Part model, mm, in its own coordinate system. Face numbers are marked on the shaded views. Coordinates: 2 decimals unless noted, no trailing zeros. Loops run counter-clockwise (first coordinate to the right, second up) from the corner with the lowest first, then second, coordinate; pieces in that order, holes last. Notation, with made-up numbers: (36.25, 81.25) - (52.25, 81.25) arc R23 cw to (52.25, 114.25) - close; hole circle Ø9 at (-22.5, 74). An arc over 180 degrees is marked (long way). Use a Markdown table: item, result. Add a question column.
1) Pull direction Z, two halves, no side cores. Call the marked faces 1, 2 and 3: +Z half, -Z half, draft (parallel to the pull), parting line (faces both ways), or undercut.
2) Drop flat-ended pins along their axis: P1, Ø1, axis at x = 0, z = 0, coming from the +Y side; P2, Ø1, axis at y = -4, z = -1, coming from the -X side; P3, Ø2, axis at x = -0.5, y = -3, coming from the -Z side. Give the stop position or say it passes through.
3) Band-saw the part on A-A (y = -3.25). Give the cut face in (x, z).
4) Probe probe 1 along Y at (x, z) = (-0.1, -0.65); probe 2 along Y at (x, z) = (1.5, 0.5); probe 3 along X at (y, z) = (0.5, 0.05). List the from-to ranges inside material, lowest first. Write a range as [from, to].
from build123d import *

# Parameters (mm, degrees)
CUT_EXTRUDE1_DEPTH = 0.75
FILLET1_R          = 0.125


with BuildPart() as part:
    # Sketch1 → Revolve1 (revolve)
    with BuildSketch(Plane(origin=(0, 0, 0), x_dir=(0, 0, -1), z_dir=(1, 0, 0)), mode=Mode.PRIVATE) as revolve1_sk:
        with BuildLine():
            Line((0, 1.5), (-1.75, 1.5))
            ThreePointArc((-1.75, 1.5), (-2.334912942, 0.942930354), (-2.75, 0.25))
            Line((-2.75, 0.25), (-2.605662433, 0))
            Line((-2.605662433, 0), (-1.5, 0))
            Line((-1.5, 0), (-1.5, -6))
            Line((-1.5, -6), (0, -6))
            Line((0, -6), (0, 1.5))
        make_face()
    revolve(revolve1_sk.sketch.rotate(Axis((0, -6, 0), (0, 1, 0)), 180), axis=Axis((0, -6, 0), (0, 1, 0)))

    # Sketch2 → Cut-Extrude1 (cut)
    with BuildSketch(Plane(origin=(0, 1.5, 0), x_dir=(1, 0, 0), z_dir=(0, 1, 0))):
        Polygon((0, 1.154700538), (-1, 0.577350269), (-1, -0.577350269), (0, -1.154700538), (1, -0.577350269), (1, 0.577350269), align=None)
    extrude(amount=-CUT_EXTRUDE1_DEPTH, mode=Mode.SUBTRACT)

    # Fillet1
    fillet1_edges = [part.edges().sort_by_distance(p)[0] for p in [
        (0.5, 1.5, -0.866025404),
        (-0.5, 1.5, -0.866025404),
        (-1, 1.5, 0),
        (-0.5, 1.5, 0.866025404),
        (0.5, 1.5, 0.866025404),
        (1, 1.5, 0),
        (0, 1.5, 1.75),
    ]]
    fillet(fillet1_edges, radius=FILLET1_R)


solid = part.part
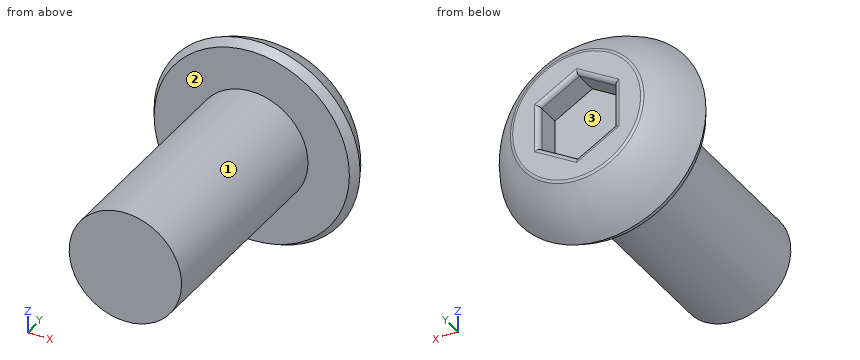
Answer block:
| question | item | result |
|---|---|---|
| 1 | face 1 | parting line |
| 1 | face 2 | draft |
| 1 | face 3 | undercut |
| 2 | P1 | y = 0.75 |
| 2 | P2 | x = -1.41 |
| 2 | P3 | z = -1.5 |
| 3 | outline | circle Ø3 at (0, 0) |
| 4 | probe 1 | [-6, 0.75] |
| 4 | probe 2 | [0, 1.5] |
| 4 | probe 3 | [-2.63, 2.63] |
